Part model, mm, in its own coordinate system. A direction names the side the tool comes from. Round coordinates to 2 decimals unless told otherwise and drop trailing zeros. Loops run counter-clockwise (first coordinate to the right, second up) from the corner with the lowest first, then second, coordinate; pieces in that order, holes last.
Autodesk Inventor part; units mm, degrees
ref_plane "YZ Plane" through (0, 0, 0) normal (1, 0, 0) x (0, 1, 0)
ref_plane "XZ Plane" through (0, 0, 0) normal (0, 1, 0) x (-1, 0, 0)
ref_plane "XY Plane" through (0, 0, 0) normal (0, 0, 1) x (1, 0, 0)
sketch "Sketch1" plane through (0, 0, 0) normal (0, 0, 1) x (1, 0, 0)
  circle A0 centre (12, 30.5) radius 7
  circle A1 centre (12, 10.5) radius 7
  line L0 (5, 23.5) -> (22.5, 23.5)
  line L1 (22.5, 23.5) -> (22.5, 17.5)
  line L2 (22.5, 17.5) -> (5, 17.5)
  line L3 (5, 17.5) -> (5, 23.5)
  line L4 (0, 41) -> (5, 41)
  line L5 (5, 41) -> (5, 0)
  line L6 (5, 0) -> (0, 0)
  line L7 (0, 0) -> (0, 41)
  circle A2 centre (12, 10.5) radius 2.6
  circle A3 centre (12, 30.5) radius 2.6
  circle A4 centre (12, 30.5) radius 10.5
  circle A5 centre (12, 10.5) radius 10.5
  line L8 (5, 41) -> (12, 41)
  line L9 (22.5, 23.5) -> (22.5, 30.5)
  line L10 (22.5, 17.5) -> (22.5, 10.5)
  line L11 (5, 0) -> (12, 0)
  line L12 (12, 10.5) -> (12, 0)
  line L13 (12, 10.5) -> (22.5, 10.5)
  line L14 (12, 30.5) -> (12, 41)
  line L15 (12, 30.5) -> (22.5, 30.5)
  point P0 (5, 17.5)
  point P1 (5, 23.5)
  point P2 (5, 10.5)
  point P3 (12, 17.5)
  point P4 (5, 30.5)
  point P5 (12, 23.5)
  point P6 (19, 10.5)
  point P7 (12, 3.5)
  point P8 (19, 30.5)
  point P9 (12, 37.5)
  dimension "d0" = 20
  dimension "d1" = 14
  dimension "d2" = 5.2
  dimension "d3" = 5.2
  dimension "d6" = 3.5
  dimension "d13" = 5
extrude "Extrusion1" add sketch "Sketch1" against normal blind 7.5 contours A0 L14 A4 L15 | L0 L5 A0 | L0 A4 A5 L3 | L5 L3 A4 | L0 L1 L2 A5 A4 | A4 L3 A5 L5 L6 L7 L4 | A4 A5 L3 | A5 L2 L3 A4 | A4 A5 | L3 L5 A5 | A5 L12 A1 L13 | L2 A1 L5
extrude "Extrusion2" add sketch "Sketch1" along normal blind 4 contours L15 A3 L14 A0 | L15 A4 L0 A0 | A0 L14 A3 L15 | A0 L14 A4 L15 | A0 L5 A4 L14 | L0 L5 A0 | L0 A4 A5 L3 | L9 L0 A4 | L5 L3 A4 | A4 L5 L8 | L0 L1 L2 A5 A4 | A4 L3 A5 L5 L6 L7 L4 | A4 A5 L3 | A5 L2 L3 A4 | A4 A5 | L10 A5 L2 | L3 L5 A5 | A5 L13 A1 L2 | A5 L12 A1 L13 | L2 A1 L5 | A5 L11 L5 | L5 A1 L12 A5 | A1 L13 A2 L12 | A1 L12 A2 L13
sketch "Sketch2" plane through (0, 0, 4) normal (0, 0, 1) x (1, 0, 0)
  line L0 (12, 41) -> (0, 41)
  line L1 (0, 41) -> (0, 0)
  line L2 (0, 0) -> (12, 0)
  arc A0 (12, 0) -> (22.5, 10.5) centre (12, 10.5) ccw
  line L3 (22.5, 10.5) -> (22.5, 30.5)
  arc A1 (22.5, 30.5) -> (12, 41) centre (12, 30.5) ccw
  circle A2 centre (12, 10.5) radius 2.6
  circle A3 centre (12, 30.5) radius 2.6
  arc A4 (22.5, 30.5) -> (12, 41) centre (12, 30.5) ccw
  line L4 (12, 41) -> (0, 37.1888)
  line L5 (5, 0) -> (12, 0)
  line L6 (12, 0) -> (0, 3.8112)
  dimension "d14" = 17.62
extrude "Extrusion3" cut sketch "Sketch2" against normal through all contours L4 L1 L0 | L6 L2 L1
properties part number "XZ Bearing Cage"
1) Slice it at D-D, the plane y = 12.5. Give the cut face in (x, z).
Values:
outline: (0, -7.5) - (5.29, -7.5) - (5.29, 0) - (10.34, 0) - (10.34, 4) - (0, 4) - close; (13.66, 0) - (22.5, 0) - (22.5, 4) - (13.66, 4) - close
2) Tool access for faces 4 (the face through (7, 25.6, -3.7)), 5 (the face through (12, 2, -4)), 6 (the face through (17, 35.4, -3.7)), 7 (the face through (14.4, 31.5, 2)), 8 (the face through (21, 10.5, -4)): list every direction of +Z, -Z, +X, -X, +Y, -Y with a clear straight run to the whole face (end or side of a thin tool).
Values:
face 4: -Z, +X, +Y
face 5: -Z, -Y
face 6: -Z
face 7: +Z, -Z
face 8: -Z, +X
3) Slice it at B-B, the plane x = 13. Give the cut face in (y, z).
Values:
outline: (0.05, -7.5) - (3.57, -7.5) - (3.57, 0) - (8.1, 0) - (8.1, 4) - (0.05, 4) - close; (12.9, 0) - (17.5, 0) - (17.5, -7.5) - (23.5, -7.5) - (23.5, 0) - (28.1, 0) - (28.1, 4) - (12.9, 4) - close; (32.9, 0) - (37.43, 0) - (37.43, -7.5) - (40.95, -7.5) - (40.95, 4) - (32.9, 4) - close
4) Slice it at A-A, the plane z = -3. Give the cut face in (x, y), then the cut area to 3 significant figures.
Values:
outline: (0, 3.81) - (5, 2.22) - (5, 10.5) arc R7 cw to (12, 17.5) - (22.5, 17.5) - (22.5, 23.5) - (12, 23.5) arc R7 cw to (5, 30.5) - (5, 38.78) - (0, 37.19) - close; (12, 0) arc R10.5 ccw to (22.5, 10.5) - (19, 10.5) arc R7 cw to (12, 3.5) - close; (12, 37.5) arc R7 cw to (19, 30.5) - (22.5, 30.5) arc R10.5 ccw to (12, 41) - close
area: 397 mm2
5) Drop flat-ended pins along their axis: pin 1 Ø4 at (x, y) = (12, 10.5) entering from -Z; pin 2 Ø2 at (y, z) = (6.5, -5.5) entering from +X; pin 3 Ø2 at (y, z) = (34, -4) entering from +X; pin 4 Ø2 at (x, z) = (5.5, 1.5) entering from -Y. Give the stop position or say it passes through.
Values:
pin 1: passes through
pin 2: stops at x = 22.06
pin 3: stops at x = 22.2
pin 4: stops at y = 1.75
6) Wall check: line 1 along Y through (x, z) = (12, 2.9); line 2 along X through (y, z) = (10.5, 2.7); line 3 along Y through (x, z) = (13.75, -5.25). Give the ranges that are in metal, low to high.
Values:
line 1: y = 0 to 7.9, 13.1 to 27.9, 33.1 to 41
line 2: x = 0 to 9.4, 14.6 to 22.5
line 3: y = 0.15 to 3.72, 17.5 to 23.5, 37.28 to 40.85
7) Mould opens along Y. For faces 1 (the face through (17, 23.5, -4)), 2 (the face through (7.1, 15.5, -3.7)), 3 (the face through (5, 35, -4)) say: released by +Y, released by -Y, zero draft, split by the parting line, or undercut.
Values:
face 1: undercut
face 2: released by -Y
face 3: zero draft
8) Slice it at C-C, the plane z = 2. Give the cut face in (x, y), then the cut area to 3 significant figures.
Values:
outline: (0, 3.81) - (12, 0) arc R10.5 ccw to (22.5, 10.5) - (22.5, 30.5) arc R10.5 ccw to (12, 41) - (0, 37.19) - close; hole circle Ø5.2 at (12, 10.5); hole circle Ø5.2 at (12, 30.5)
area: 787 mm2
